```python
from build123d import *

# Parameters (mm, degrees)
SKETCH2_R           = 7
SKETCH2_R_2         = 4.5
CUT_EXTRUDE1_DEPTH  = 0.5
CHAMFER3_SIZE       = 1
BOSS_EXTRUDE1_START = 2
SKETCH3_R           = 4.5
SKETCH3_R_2         = 2.505
BOSS_EXTRUDE1_DEPTH = 2
CHAMFER4_SIZE       = 2
CHAMFER4_SIZE_2     = 3.464101615
SKETCH4_R           = 9.505
SKETCH4_R_2         = 2.505
BOSS_EXTRUDE2_DEPTH = 3
FILLET1_R           = 0.5
FILLET2_R           = 3
CHAMFER5_SIZE       = 0.6


with BuildPart() as part:
    # Sketch1 → Revolve1 (revolve)
    with BuildSketch(Plane.XY, mode=Mode.PRIVATE) as revolve1_sk:
        with BuildLine():
            Line((-3, -9.505), (-3, -2.505))
            Line((-3, -2.505), (3, -2.505))
            Line((3, -2.505), (3, -9.505))
            ThreePointArc((3, -9.505), (0, -8.150751311), (-3, -9.505))
        make_face()
    revolve(revolve1_sk.sketch.rotate(Axis((0, 0, 0), (-1, 0, 0)), 270), axis=Axis((0, 0, 0), (-1, 0, 0)))

    # Sketch2 → Cut-Extrude1 (cut)
    with BuildSketch(Plane(origin=(3, 0, 0), x_dir=(0, 0, -1), z_dir=(1, 0, 0))):
        Circle(SKETCH2_R)
        Circle(SKETCH2_R_2, mode=Mode.SUBTRACT)
    extrude(amount=-CUT_EXTRUDE1_DEPTH, mode=Mode.SUBTRACT)

    # Chamfer3
    # the kernel refuses this chamfer: 1 mm, written as the material it takes off along each edge
    with BuildSketch(Plane(origin=(3, 0, 0), x_dir=(0, 0, -1), z_dir=(0, -1, 0))) as chamfer3_piece_1_section:
        Polygon((7 + CHAMFER3_SIZE, 0), (7, -CHAMFER3_SIZE), (7, 0), align=None)
    chamfer3_piece_1 = revolve(axis=Axis((3, 0, 0), (1, 0, 0)), mode=Mode.PRIVATE)
    chamfer3_piece_1 = split(chamfer3_piece_1, bisect_by=Plane(origin=(2.5, 0, 7.745273701), z_dir=(1, 0, 0)), keep=Keep.TOP, mode=Mode.PRIVATE)
    add(chamfer3_piece_1, mode=Mode.SUBTRACT)

    # Sketch3 → Boss-Extrude1 (add)
    with BuildSketch(Plane(origin=(3, 0, 0), x_dir=(0, 0, -1), z_dir=(1, 0, 0)).offset(BOSS_EXTRUDE1_START)):
        Circle(SKETCH3_R)
        Circle(SKETCH3_R_2, mode=Mode.SUBTRACT)
    extrude(amount=-BOSS_EXTRUDE1_DEPTH)

    # Chamfer4
    # the kernel refuses this chamfer: 3.464101615, 2 mm, written as the material it adds along each edge
    with BuildSketch(Plane(origin=(2.5, 0, 0), x_dir=(0, 0, -1), z_dir=(0, -1, 0))) as chamfer4_piece_1_section:
        Polygon((4.5 + CHAMFER4_SIZE, 0), (4.5, CHAMFER4_SIZE_2), (4.5, 0), align=None)
    chamfer4_piece_1 = revolve(axis=Axis((2.5, 0, 0), (1, 0, 0)), mode=Mode.PRIVATE)
    chamfer4_piece_1 = split(chamfer4_piece_1, bisect_by=Plane(origin=(5, 0, 5.770731059), z_dir=(-1, 0, 0)), keep=Keep.TOP, mode=Mode.PRIVATE)
    add(chamfer4_piece_1)

    # Sketch4 → Boss-Extrude2 (add)
    with BuildSketch(Plane.ZY.offset(3)):
        Circle(SKETCH4_R)
        with Locations(Location((0, 0, 0), (0, 0, 180))):
            Circle(SKETCH4_R_2, mode=Mode.SUBTRACT)
    extrude(amount=BOSS_EXTRUDE2_DEPTH)

    # Fillet1
    fillet1_edges = [part.edges().sort_by_distance(p)[0] for p in [
        (3, 0, 9.505),
    ]]
    fillet(fillet1_edges, radius=FILLET1_R)

    # Fillet2
    fillet2_edges = [part.edges().sort_by_distance(p)[0] for p in [
        (-3, -9.505, 0),
    ]]
    fillet(fillet2_edges, radius=FILLET2_R)

    # Chamfer5
    chamfer5_edges = [part.edges().sort_by_distance(p)[0] for p in [
        (-6, 0, -9.505),
        (-6, 0, 2.505),
    ]]
    chamfer(chamfer5_edges, length=CHAMFER5_SIZE)


solid = part.part
```
Verification items for the finished model (mm, model axes). Coordinates: 2 decimals unless noted, no trailing zeros. Write each loop counter-clockwise with the first axis right and the second up, starting at its lowest first coordinate (ties: lowest second). Pieces come first, ordered by that corner, then holes. Notation, with made-up numbers: M 54,11.25 L 83,11.25 A15 ccw 83,16.25 Z; hole C 11,81 d9. An arc over 180 degrees is marked long. Answer as a JSON object with one key per item and string values. Group by question number.
(1) Gauge pin test, flat ends, axial feed: pin 1 (3 mm diameter, centred on x = -4, z = 5, fed in from +Y); pin 2 (3 mm diameter, centred on y = 0, z = 0, fed in from -X); pin 3 (6 mm diameter, centred on x = -3.5, z = -5, fed in from +Y); pin 4 (1 mm diameter, centred on x = 2, y = 2.5, fed in from -Z). Record the tip position at first contact, or that the pin passes through.
(2) Release check for a two-part mould opening along Y. For faces 1 (the face through (2.5, -3, -6)), 2 (the face through (5, 2, -2)), 3 (the face through (-4.76, 2.855, 9.066)) record: +Y half, -Y half, draft (parallel to the pull), parting line (faces both ways), or undercut.
(3) Cross-section at B-B, the plane x = -0.5. Record the cut outline in (y, z) (3 decimals), and give its area (3 significant figures).
(4) Cross-section at A-A, the plane x = -4.5. Record the cut outline in (y, z) (3 decimals), and give its area (3 significant figures).
(5) Material ranges on line 1 (Y direction, x = -4, z = 0) (3 decimals); line 2 (Y direction, x = 2.75, z = 2.75); line 3 (X direction, y = -6.5, z = 3.25), recorded low to high.
Reply:
{
 "1": {"pin 1": "y = 8.84", "pin 2": "through", "pin 3": "y = 9.28", "pin 4": "z = -8.62"},
 "2": {"face 1": "undercut", "face 2": "draft", "face 3": "parting line"},
 "3": {"outline": "C 0,0 d16.364; hole C 0,0 d5.01", "area": "191 mm²"},
 "4": {"outline": "C 0,0 d19.01; hole C 0,0 d5.01", "area": "264 mm²"},
 "5": {"line 1": "-9.502 to -2.505, 2.505 to 9.502", "line 2": "-8.4 to -7.25, -5.73 to 5.73, 7.25 to 8.4", "line 3": "-6 to 2.5"}
}
